from build123d import *

# Parameters (mm, degrees)
ESQUISSE1_R             = 0.25
BOSS_EXTRU_1_DEPTH      = 5
ESQUISSE2_W             = 5
ESQUISSE2_H             = 5
ENL_V_MAT_EXTRU_1_DEPTH = 5


with BuildPart() as part:
    # Esquisse1 → Boss.-Extru.1 (new body)
    with BuildSketch(Plane.XY):
        with BuildLine():
            Line((0, 80), (40, 80))
            Line((40, 80), (40, 72.5))
            ThreePointArc((40, 72.5), (7.5, 40), (40, 7.5))
            Line((40, 7.5), (40, 0))
            Line((40, 0), (0, 0))
            Line((0, 0), (0, 80))
        make_face()
        with Locations((2.018546053, 59.069849399)):
            Circle(ESQUISSE1_R, mode=Mode.SUBTRACT)
        with Locations((7.641889366, 67.553632723)):
            Circle(ESQUISSE1_R, mode=Mode.SUBTRACT)
        with Locations((9.9479618, 70.0520382)):
            Circle(ESQUISSE1_R, mode=Mode.SUBTRACT)
        with Locations((3.664453699, 62.04491041)):
            Circle(ESQUISSE1_R, mode=Mode.SUBTRACT)
        with Locations((5.542908841, 64.878883995)):
            Circle(ESQUISSE1_R, mode=Mode.SUBTRACT)
        with Locations(Location((20.930150601, 77.981453947, 0), (0, 0, 180))):
            Circle(ESQUISSE1_R, mode=Mode.SUBTRACT)
        with Locations(Location((17.95508959, 76.335546301, 0), (0, 0, 180))):
            Circle(ESQUISSE1_R, mode=Mode.SUBTRACT)
        with Locations(Location((15.121116005, 74.457091159, 0), (0, 0, 180))):
            Circle(ESQUISSE1_R, mode=Mode.SUBTRACT)
        with Locations(Location((12.446367277, 72.358110634, 0), (0, 0, 180))):
            Circle(ESQUISSE1_R, mode=Mode.SUBTRACT)
        with Locations((12.446367277, 7.641889366)):
            Circle(ESQUISSE1_R, mode=Mode.SUBTRACT)
        with Locations((15.121116005, 5.542908841)):
            Circle(ESQUISSE1_R, mode=Mode.SUBTRACT)
        with Locations((17.95508959, 3.664453699)):
            Circle(ESQUISSE1_R, mode=Mode.SUBTRACT)
        with Locations((20.930150601, 2.018546053)):
            Circle(ESQUISSE1_R, mode=Mode.SUBTRACT)
        with Locations(Location((5.542908841, 15.121116005, 0), (0, 0, 180))):
            Circle(ESQUISSE1_R, mode=Mode.SUBTRACT)
        with Locations(Location((3.664453699, 17.95508959, 0), (0, 0, 180))):
            Circle(ESQUISSE1_R, mode=Mode.SUBTRACT)
        with Locations(Location((9.9479618, 9.9479618, 0), (0, 0, 180))):
            Circle(ESQUISSE1_R, mode=Mode.SUBTRACT)
        with Locations(Location((7.641889366, 12.446367277, 0), (0, 0, 180))):
            Circle(ESQUISSE1_R, mode=Mode.SUBTRACT)
        with Locations(Location((2.018546053, 20.930150601, 0), (0, 0, 180))):
            Circle(ESQUISSE1_R, mode=Mode.SUBTRACT)
    extrude(amount=BOSS_EXTRU_1_DEPTH)

    # Esquisse2 → Enlèv. mat.-Extru.1 (cut)
    with BuildSketch(Plane.XY.offset(5)):
        with Locations((2.5, 2.5)):
            Rectangle(ESQUISSE2_W, ESQUISSE2_H)
        with Locations((37.5, 2.5)):
            Rectangle(ESQUISSE2_W, ESQUISSE2_H)
        with Locations((37.5, 77.5)):
            Rectangle(ESQUISSE2_W, ESQUISSE2_H)
        with Locations((2.5, 77.5)):
            Rectangle(ESQUISSE2_W, ESQUISSE2_H)
    extrude(amount=-ENL_V_MAT_EXTRU_1_DEPTH, mode=Mode.SUBTRACT)


solid = part.part
Input: part model. Units: mm. Frame: model coordinates. A direction names the side the tool comes from. Coordinates: 2 decimals unless noted, no trailing zeros. Loops run counter-clockwise (first coordinate to the right, second up) from the corner with the lowest first, then second, coordinate; pieces in that order, holes last.
Q1. Material intervals for line 1 (X direction, y = 5.5, z = 0.75); line 2 (Y direction, x = 13.5, z = 1.3); line 3 (X direction, y = 27, z = 1.7), sorted ascending.
Q2. Draft query along Y for faces 6 (the face through (20, 0, 2)), 7 (the face through (7.508, 40.715, 2.465)), 8 (the face through (35, 2, 3)). Return one class per face: +Y half, -Y half, draft (parallel to the pull), parting line (faces both ways), or undercut.
Q3. Cut plane B-B (z = 3.25). Give the number of separate pieces and of enclosed holes in the cut face, then the cut area to 3 significant figures.
Q4. Cut plane D-D (y = 40). Output: boundary loops of the cut face in (x, z).
Q5. Set-up query: faces 1 (the face through (35, 77, 3)), 2 (the face through (2, 75, 3)), 3 (the face through (2, 5, 3)), 4 (the face through (7, 41, 5)), 5 (the face through (37, 5, 3)). Return all of +Z, -Z, +X, -X, +Y, -Y with unobstructed straight access to the full face (end or side cutting, diameter ignored); none if empty.
Q6. Contact query for flat-ended pins moving along their axis: pin 1 (1.5 mm diameter, centred on x = 38.5, z = 3, fed in from -Y); pin 2 (2.5 mm diameter, centred on x = 3.5, z = 2.5, fed in from +Y); pin 3 (2.5 mm diameter, centred on y = 78, z = 2.5, fed in from +X). Output: stop coordinate, or through.
Q7. Cut plane A-A (x = 24). Output: boundary loops of the cut face in (y, z).
Q8. Cut plane C-C (y = 52.5). Output: boundary loops of the cut face in (x, z), then the cut area to 3 significant figures.
Working result:
1. line 1: x = 0 to 14.87, 15.37 to 40
1. line 2: y = 0 to 21.19, 58.81 to 80
1. line 3: x = 0 to 10.21
2. face 6: -Y half
2. face 7: undercut
2. face 8: draft
3. separate pieces: 1
3. enclosed holes: 18
3. area: 1,440 mm2
4. outline: (0, 0) - (7.5, 0) - (7.5, 5) - (0, 5) - close
5. face 1: +Z, -Z, +X, +Y
5. face 2: +Z, -Z, -X, +Y
5. face 3: +Z, -Z, -X, -Y
5. face 4: +Z, +X, -X, +Y, -Y
5. face 5: +Z, -Z, +X, -Y
6. pin 1: stops at y = 5
6. pin 2: stops at y = 75
6. pin 3: stops at x = 35
7. outline: (0, 0) - (11.71, 0) - (11.71, 5) - (0, 5) - close; (68.29, 0) - (80, 0) - (80, 5) - (68.29, 5) - close
8. outline: (0, 0) - (10, 0) - (10, 5) - (0, 5) - close
8. area: 50.0 mm2
